from build123d import *

# Parameters (mm, degrees)
SKETCH1_W           = 50
SKETCH1_H           = 30
BOSS_EXTRUDE1_DEPTH = 20
SKETCH2_R           = 5
SKETCH2_R_2         = 5.015568952
BOSS_EXTRUDE3_DEPTH = 20
SKETCH3_R           = 0.75
BOSS_EXTRUDE4_DEPTH = 10


with BuildPart() as part:
    # Sketch1 → Boss-Extrude1 (new body)
    with BuildSketch(Plane.XY):
        with Locations((-92.348484848, 31.333080808)):
            Rectangle(SKETCH1_W, SKETCH1_H)
    extrude(amount=BOSS_EXTRUDE1_DEPTH)

    # Sketch2 → Boss-Extrude3 (add)
    with BuildSketch(Plane.XZ.offset(-16.333080808)):
        with Locations(Location((-108.512795062, 10.404107755, 0), (0, 0, 90))):
            Circle(SKETCH2_R)
        with Locations(Location((-78.512795062, 10.404107755, 0), (0, 0, 90))):
            Circle(SKETCH2_R_2)
    extrude(amount=BOSS_EXTRUDE3_DEPTH)

    # Sketch3 → Boss-Extrude4 (add)
    with BuildSketch(Plane.XY.offset(20)):
        with Locations((-112.98809036, 39.90814541)):
            Circle(SKETCH3_R)
        with Locations((-71.988091026, 39.915535227)):
            Circle(SKETCH3_R)
        with Locations(Location((-71.988091026, 24.378479398, 0), (0, 0, 180))):
            Circle(SKETCH3_R)
        with Locations(Location((-112.98809036, 24.385869214, 0), (0, 0, 180))):
            Circle(SKETCH3_R)
    extrude(amount=BOSS_EXTRUDE4_DEPTH)


solid = part.part
Check sheet for the modelled part. Datum: model origin and axes. Units: mm. A direction names the side the tool comes from. Round coordinates to 2 decimals unless told otherwise and drop trailing zeros. Write each loop counter-clockwise with the first axis right and the second up, starting at its lowest first coordinate (ties: lowest second). Pieces come first, ordered by that corner, then holes. Notation, with made-up numbers: (-11, -3.5) - (22, -3.5) arc R19 cw to (22, 29.5) - close; hole circle Ø2 at (33.5, 34.5). An arc over 180 degrees is marked (long way). Return JSON: item names as keys, results as strings.
Q1. Cross-section at B-B (x = -111.5). Record the boundary of the cut face in (y, z), then the cut area to 3 significant figures.
Returned:
{"outline": "(-3.67, 6.39) - (16.33, 6.39) - (16.33, 0) - (46.33, 0) - (46.33, 20) - (16.33, 20) - (16.33, 14.41) - (-3.67, 14.41) - close", "area": "760 mm²"}
Q2. Scan lines: L1, parallel to Z at x = -89.5, y = 28.5; L2, parallel to X at y = 9, z = 9.25; L3, parallel to Y at x = -87, z = 1.75. Record each from-to range of solid material in increasing order. Write a range as from..to.
Returned:
{"L1": "z = 0..20", "L2": "x = -113.38..-103.65, -83.39..-73.63", "L3": "y = 16.33..46.33"}
Q3. Depth check by flat-ended pin: P1, Ø8, axis at x = -107, y = 8, coming from the -Z side; P2, Ø8, axis at x = -84.5, y = 19.5, coming from the +Z side; P3, Ø5, axis at x = -93, z = 19, coming from the -Y side. Enter the tip coordinate at first touch or a pass-through.
Returned:
{"P1": "stops at z = 5.4", "P2": "stops at z = 20", "P3": "stops at y = 16.33"}
Q4. Cross-section at D-D (z = 21.25). Record the boundary of the cut face in (x, y), then the cut area to 3 significant figures.
Returned:
{"outline": "circle Ø1.5 at (-112.99, 24.39); circle Ø1.5 at (-112.99, 39.91); circle Ø1.5 at (-71.99, 24.38); circle Ø1.5 at (-71.99, 39.92)", "area": "7.07 mm²"}
Q5. Access from +Z, -Z, +X, -X, +Y, -Y to the whole of each face (thin tool, end or side, straight path). Record for faces 5 (the cylindrical face through (-82.74, 6.47, 13.1)), 6 (the cylindrical face through (-112.295, 39.621, 24.93)), 7 (the flat face through (-93, 32, 0)).
Returned:
{"face 5": "-Y", "face 6": "+Z", "face 7": "-Z, +X, -X, +Y, -Y"}
Q6. Cross-section at A-A (z = 10.25). Record the boundary of the cut face in (x, y), then the cut area to 3 significant figures.
Returned:
{"outline": "(-117.35, 16.33) - (-113.51, 16.33) - (-113.51, -3.67) - (-103.52, -3.67) - (-103.52, 16.33) - (-83.53, 16.33) - (-83.53, -3.67) - (-73.5, -3.67) - (-73.5, 16.33) - (-67.35, 16.33) - (-67.35, 46.33) - (-117.35, 46.33) - close", "area": "1,900 mm²"}
Q7. Draft check along X on faces 1 (the flat face through (-93, 16.333, 10)), 2 (the cylindrical face through (-72.737, 39.949, 24.93)), 3 (the flat face through (-67.348, 31, 10)), 4 (the flat face through (-72, 40, 30)). Enter one of: released by +X, released by -X, zero draft, split by the parting line, or undercut.
Returned:
{"face 1": "undercut", "face 2": "undercut", "face 3": "released by +X", "face 4": "zero draft"}
Q8. Cross-section at C-C (y = 17.5). Record the boundary of the cut face in (x, z), then the cut area to 3 significant figures.
Returned:
{"outline": "(-117.35, 0) - (-67.35, 0) - (-67.35, 20) - (-117.35, 20) - close", "area": "1,000 mm²"}
